The listing builds one solid part. Answer for the finished solid, in the listing's coordinates (mm). A direction names the side the tool comes from. Round coordinates to 2 decimals unless told otherwise and drop trailing zeros. Write each loop counter-clockwise with the first axis right and the second up, starting at its lowest first coordinate (ties: lowest second). Pieces come first, ordered by that corner, then holes.
Item 1: Find the intervals of material crossed by probe 1 along X at (y, z) = (2.25, -8.75); probe 2 along X at (y, z) = (-0.75, -7.75); probe 3 along Y at (x, z) = (1.75, -7.75), in increasing order.
Item 2: For a pull along Y with two mould halves and no side action, classify faces 5 (the face through (5, -1.5, -9)), 6 (the face through (0.5, 2, -6)), 7 (the face through (5, -1, -4.969)), 8 (the face through (1, 2.5, -6)) as +Y half, -Y half, draft (parallel to the pull), parting line (faces both ways), or undercut.
Item 3: Find section D-D on y = 2.25. Give the vertices of the cut face in (x, z), then the cut area to 3 significant figures.
Item 4: A tool of negligible diameter and unlimited length cuts with its end or side. For faces 1 (the face through (-5, -1, -4.969)), 2 (the face through (-5, -1.5, -9)), 3 (the face through (-1, 1, -6)), 4 (the face through (4.335, -1, -9)), from which of +Z, -Z, +X, -X, +Y, -Y can it reach the whole face along a straight path? Write none if from no direction.
Item 5: Each of these flat-tipped pins is pushed along its axis until it touches: pin 1 (0.5 mm diameter, centred on x = -4.5, y = -0.5, fed in from +Z); pin 2 (0.8 mm diameter, centred on x = 1, z = -4, fed in from -Y). Where does it stop, or does it pass through?
Item 6: Find section A-A on x = -1.5. Give the vertices of the cut face in (y, z), then the cut area to 3 significant figures.
Item 7: Find section C-C on z = -10.75. Give the vertices of the cut face in (x, y).
Item 8: Find section B-B on y = -1. Give the vertices of the cut face in (x, z).
```python
from build123d import *

# Parameters (mm, degrees)
SKETCH_1_W          = 10.8
SKETCH_1_H          = 12.8
EXTRUDE_1_DEPTH     = 5
SKETCH_2_W          = 1.5
SKETCH_2_H          = 1.5
CUT_EXTRUDE_1_DEPTH = 13.8
SKETCH_3_W          = 0.979411712
SKETCH_3_H          = 7.830694271
SKETCH_3_W_2        = 1.065082028
EXTRUDE_2_DEPTH     = 1.5


with BuildPart() as part:
    # 草圖1 → 填料-伸長1 (new body)
    with BuildSketch(Plane(origin=(0, 0, 0), x_dir=(1, 0, 0), z_dir=(0, 1, 0))):
        with Locations((0, 6.4)):
            Rectangle(SKETCH_1_W, SKETCH_1_H)
    extrude(amount=EXTRUDE_1_DEPTH)

    # 草圖2 → 除料-伸長1 (cut, through all)
    with BuildSketch(Plane(origin=(0, 0, -12.8), x_dir=(-1, 0, 0), z_dir=(0, 0, -1))):
        with Locations((-3.75, 1.75)):
            Rectangle(SKETCH_2_W, SKETCH_2_H)
        with Locations((-1.25, 1.75)):
            Rectangle(SKETCH_2_W, SKETCH_2_H)
        with Locations((1.25, 1.75)):
            Rectangle(SKETCH_2_W, SKETCH_2_H)
        with Locations((3.75, 1.75)):
            Rectangle(SKETCH_2_W, SKETCH_2_H)
    extrude(amount=-CUT_EXTRUDE_1_DEPTH, mode=Mode.SUBTRACT)

    # 草圖3 → 填料-伸長2 (add)
    with BuildSketch(Plane.XZ):
        with Locations((-4.910294144, -8.884652865)):
            Rectangle(SKETCH_3_W, SKETCH_3_H)
        with Locations((4.867458986, -8.884652865)):
            Rectangle(SKETCH_3_W_2, SKETCH_3_H)
    extrude(amount=EXTRUDE_2_DEPTH)


solid = part.part
```
Check values:
1. probe 1: x = -5.4 to -4.5, -3 to -2, -0.5 to 0.5, 2 to 3, 4.5 to 5.4
1. probe 2: x = -5.4 to -4.42, 4.33 to 5.4
1. probe 3: y = 0 to 1, 2.5 to 5
2. face 5: -Y half
2. face 6: undercut
2. face 7: draft
2. face 8: undercut
3. outline: (-5.4, -12.8) - (-4.5, -12.8) - (-4.5, 0) - (-5.4, 0) - close; (-3, -12.8) - (-2, -12.8) - (-2, 0) - (-3, 0) - close; (-0.5, -12.8) - (0.5, -12.8) - (0.5, 0) - (-0.5, 0) - close; (2, -12.8) - (3, -12.8) - (3, 0) - (2, 0) - close; (4.5, -12.8) - (5.4, -12.8) - (5.4, 0) - (4.5, 0) - close
3. area: 61.4 mm2
4. face 1: +Z, +X, -X, -Y
4. face 2: +Z, -Z, +X, -X, -Y
4. face 3: +Z, -Z
4. face 4: +Z, -Z, -Y
5. pin 1: stops at z = -4.97
5. pin 2: stops at y = 0
6. outline: (0, -12.8) - (1, -12.8) - (1, 0) - (0, 0) - close; (2.5, -12.8) - (5, -12.8) - (5, 0) - (2.5, 0) - close
6. area: 44.8 mm2
7. outline: (-5.4, -1.5) - (-4.42, -1.5) - (-4.42, 0) - (4.33, 0) - (4.33, -1.5) - (5.4, -1.5) - (5.4, 5) - (-5.4, 5) - close; hole (-4.5, 1) - (-3, 1) - (-3, 2.5) - (-4.5, 2.5) - close; hole (-2, 1) - (-0.5, 1) - (-0.5, 2.5) - (-2, 2.5) - close; hole (0.5, 1) - (2, 1) - (2, 2.5) - (0.5, 2.5) - close; hole (3, 1) - (4.5, 1) - (4.5, 2.5) - (3, 2.5) - close
8. outline: (-5.4, -12.8) - (-4.42, -12.8) - (-4.42, -4.97) - (-5.4, -4.97) - close; (4.33, -12.8) - (5.4, -12.8) - (5.4, -4.97) - (4.33, -4.97) - close
